Autodesk Inventor part; units mm, degrees
ref_plane "YZ Plane" through (0, 0, 0) normal (1, 0, 0) x (0, 1, 0)
ref_plane "XZ Plane" through (0, 0, 0) normal (0, 1, 0) x (-1, 0, 0)
ref_plane "XY Plane" through (0, 0, 0) normal (0, 0, 1) x (1, 0, 0)
sketch "Szkic1" plane through (0, 0, 0) normal (0, 1, 0) x (-1, 0, 0)
  line L0 (0, 0) -> (92.7, 0)
  line L1 (92.7, 0) -> (92.7, -98)
  line L2 (92.7, -98) -> (0, -98)
  line L3 (0, -98) -> (0, 0)
  line L4 (4.5, -98) -> (12.5, -98)
  line L5 (12.5, -98) -> (12.5, -90.1)
  line L6 (12.5, -90.1) -> (4.5, -90.1)
  line L7 (4.5, -90.1) -> (4.5, -98)
  line L8 (57.5, -98) -> (87.7, -98)
  line L9 (87.7, -98) -> (87.7, -78)
  line L10 (87.7, -78) -> (57.5, -78)
  line L11 (57.5, -78) -> (57.5, -98)
  line L12 (92.7, -49) -> (0, -49) construction
  line L13 (92.7, 0) -> (0, 0)
  line L14 (4.5, 0) -> (12.5, 0)
  line L15 (12.5, 0) -> (12.5, -7.9)
  line L16 (12.5, -7.9) -> (4.5, -7.9)
  line L17 (4.5, -7.9) -> (4.5, 0)
  line L18 (57.5, 0) -> (87.7, 0)
  line L19 (87.7, 0) -> (87.7, -20)
  line L20 (87.7, -20) -> (57.5, -20)
  line L21 (57.5, -20) -> (57.5, 0)
  dimension "d0" = 92.7
  dimension "d1" = 98
  dimension "d2" = 57.5
  dimension "d3" = 30.2
  dimension "d4" = 20
  dimension "d5" = 7.9
  dimension "d6" = 8
  dimension "d8" = 4.5
extrude "Wyciągnięcie proste1" add sketch "Szkic1" along normal blind 2 contours L0 L17 L16 L15 L21 L20 L19 L1 L2 L9 L10 L11 L5 L6 L7 L3
sketch "Szkic2" plane through (0, 2, 0) normal (0, 1, 0) x (1, 0, 0)
  line L0 (0, 0) -> (0, 98) construction
  line L1 (0, 49) -> (-92.7, 49) construction
  line L2 (-92.7, 98) -> (-92.7, 0) construction
  line L3 (-2.2, 49) -> (-2.2, 87.6) construction
  line L4 (-52.4, 94.75) -> (-15.8, 94.75) construction
  line L5 (-87.45, 74.6) -> (-58.85, 74.6) construction
  line L6 (-87.45, 49) -> (-87.45, 74.6) construction
  line L7 (-57.5, 78) -> (-87.7, 78) construction
  line L8 (-12.5, 98) -> (-57.5, 98) construction
  line L9 (-12.5, 90.1) -> (-12.5, 98) construction
  line L10 (-52.4, 3.25) -> (-15.8, 3.25) construction
  line L11 (-87.45, 23.4) -> (-58.85, 23.4) construction
  line L12 (-57.5, 20) -> (-87.7, 20) construction
  line L13 (-12.5, 0) -> (-57.5, 0) construction
  line L14 (-12.5, 7.9) -> (-12.5, 0) construction
  point P0 (-2.2, 10.4)
  point P1 (-50.7, 74.6)
  dimension "d11" = 2.2
  dimension "d12" = 38.6
  dimension "d13" = 3.25
  dimension "d14" = 3.3
  dimension "d15" = 36.6
  dimension "d16" = 3.4
  dimension "d17" = 5.25
  dimension "d18" = 28.6
  dimension "d26" = 42
hole "Otwór1" at (-2.2, 2, -87.6) at (-2.2, 2, -49) at (-15.8, 2, -94.75) at (-52.4, 2, -94.75) at (-58.85, 2, -74.6) at (-87.45, 2, -74.6) at (-87.45, 2, -49) at (-52.4, 2, -3.25) at (-15.8, 2, -3.25) at (-87.45, 2, -23.4) at (-58.85, 2, -23.4) at (-2.2, 2, -10.4) at (-50.7, 2, -74.6) direction (0, -1, 0) diameter 2.459 end through all
properties part number "Blacha" material "Stal"
Model file for the job. Use its own axes, mm. Round coordinates to 2 decimals unless told otherwise and drop trailing zeros. Write each loop counter-clockwise with the first axis right and the second up, starting at its lowest first coordinate (ties: lowest second). Pieces come first, ordered by that corner, then holes. Notation, with made-up numbers: (-24, 81) - (11, 81) arc R15 ccw to (11, 86) - close; hole circle Ø6 at (35, 61). An arc over 180 degrees is marked (long way). One line per item, written item: value.
(1) Cut at B-B, the plane z = -23.4. Give the cut face in (x, y), plus the area to 3 significant figures.
Values follow:
outline: (-92.7, 0) - (-88.68, 0) - (-88.68, 2) - (-92.7, 2) - close; (-86.22, 0) - (-60.08, 0) - (-60.08, 2) - (-86.22, 2) - close; (-57.62, 0) - (0, 0) - (0, 2) - (-57.62, 2) - close
area: 176 mm²
(2) Drop flat-ended pins along their axis: P1, Ø12, axis at x = -72.5, z = -13, coming from the +Y side; P2, Ø0.6, axis at x = -67, y = 1, coming from the -Z side. Give the stop position or say it passes through.
Values follow:
P1: passes through
P2: stops at z = -78
(3) Cut at C-C, the plane z = -94.75. Give the cut face in (x, y).
Values follow:
outline: (-92.7, 0) - (-87.7, 0) - (-87.7, 2) - (-92.7, 2) - close; (-57.5, 0) - (-53.63, 0) - (-53.63, 2) - (-57.5, 2) - close; (-51.17, 0) - (-17.03, 0) - (-17.03, 2) - (-51.17, 2) - close; (-14.57, 0) - (-12.5, 0) - (-12.5, 2) - (-14.57, 2) - close; (-4.5, 0) - (0, 0) - (0, 2) - (-4.5, 2) - close
(4) Two-plate mould, pull along Z, no slides. Class faces 1 (the flat face through (-46, 2, -48)), 2 (the cylindrical face through (-1.11, 0.99, -9.83)): pulls with the +Z half, pulls with the -Z half, needs draft (parallel to the pull), parting line crosses it, or undercut.
Values follow:
face 1: needs draft
face 2: undercut
(5) Cut at A-A, the plane x = -15.8. Give the cut face in (y, z), plus the area to 3 significant figures.
Values follow:
outline: (0, -98) - (2, -98) - (2, -95.98) - (0, -95.98) - close; (0, -93.52) - (2, -93.52) - (2, -4.48) - (0, -4.48) - close; (0, -2.02) - (2, -2.02) - (2, 0) - (0, 0) - close
area: 186 mm²
(6) Cut at D-D, the plane y = 1.65. Give the number of separate pieces and of enclosed holes in the cut face, plus the area to 3 significant figures.
Values follow:
separate pieces: 1
enclosed holes: 13
area: 7,690 mm²
(7) Wall check: probe 1 along X at (y, z) = (0.6, -94.75); probe 2 along X at (y, z) = (1, -74.6); probe 3 along X at (y, z) = (1.15, -49). Give the ranges that are in metal, low to high.
Values follow:
probe 1: x = -92.7 to -87.7, -57.5 to -53.63, -51.17 to -17.03, -14.57 to -12.5, -4.5 to 0
probe 2: x = -92.7 to -88.68, -86.22 to -60.08, -57.62 to -51.93, -49.47 to 0
probe 3: x = -92.7 to -88.68, -86.22 to -3.43, -0.97 to 0
